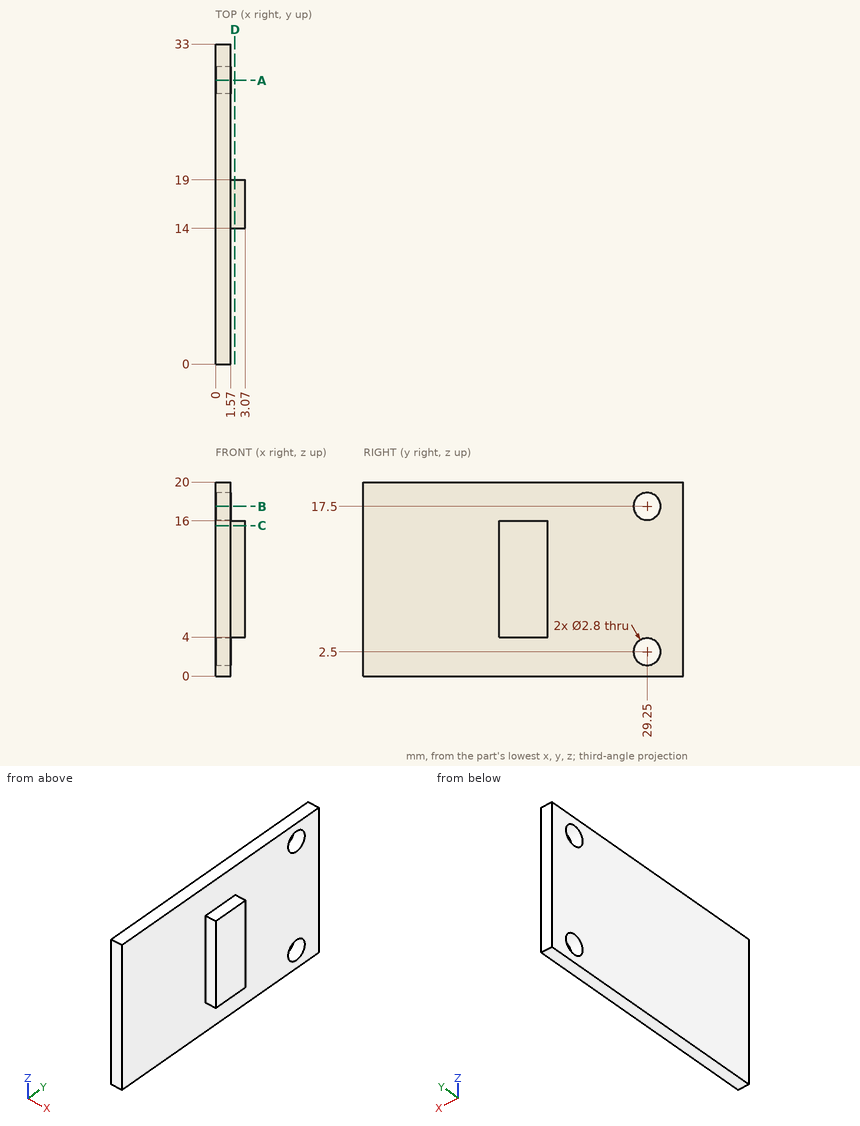
Design review of the part shown in the three views and the two pictorial views. Dimensions are in mm from the part's minimum x, y and z. Round coordinates to 2 decimals unless told otherwise and drop trailing zeros. Order: outer loops, then holes, each group sorted by start corner. A loop starts at its lowest first (then second) coordinate and runs counter-clockwise, first axis right, second up.
(1) Take a section at B-B, the plane z = 17.5. State the section outline as (x, y) points, plus the area to 3 significant figures.
Working result:
outline: (0, 0) - (1.57, 0) - (1.57, 27.85) - (0, 27.85) - close; (0, 30.65) - (1.57, 30.65) - (1.57, 33) - (0, 33) - close
area: 47.4 mm2
(2) Wall thickness on L1, parallel to Y at x = 0.4, z = 17.5; L2, parallel to X at y = 10.5, z = 14; L3, parallel to Y at x = 2.4, z = 13.25: over which ranges is each line inside the solid? List them lowest first.
Working result:
L1: y = 0 to 27.85, 30.65 to 33
L2: x = 0 to 1.57
L3: y = 14 to 19
(3) For P1, Ø0.5, axis at x = 2.5, y = 16.5, coming from the +Z side; P2, Ø0.5, axis at x = 2.5, y = 15.5, coming from the -Z side; P3, Ø3, axis at y = 12, z = 12.5, coming from the +X side, all flat-tipped, find the tip position at first contact; note any pin that passes through.
Working result:
P1: stops at z = 16
P2: stops at z = 4
P3: stops at x = 1.57
(4) Take a section at A-A, the plane y = 29.25. State the section outline as (x, z) points.
Working result:
outline: (0, 0) - (1.57, 0) - (1.57, 1.1) - (0, 1.1) - close; (0, 3.9) - (1.57, 3.9) - (1.57, 16.1) - (0, 16.1) - close; (0, 18.9) - (1.57, 18.9) - (1.57, 20) - (0, 20) - close
(5) Take a section at C-C, the plane z = 15.5. State the section outline as (x, y) points, plus the area to 3 significant figures.
Working result:
outline: (0, 0) - (1.57, 0) - (1.57, 14) - (3.07, 14) - (3.07, 19) - (1.57, 19) - (1.57, 33) - (0, 33) - close
area: 59.3 mm2
(6) Take a section at D-D, the plane x = 2. State the section outline as (y, z) points.
Working result:
outline: (14, 4) - (19, 4) - (19, 16) - (14, 16) - close
